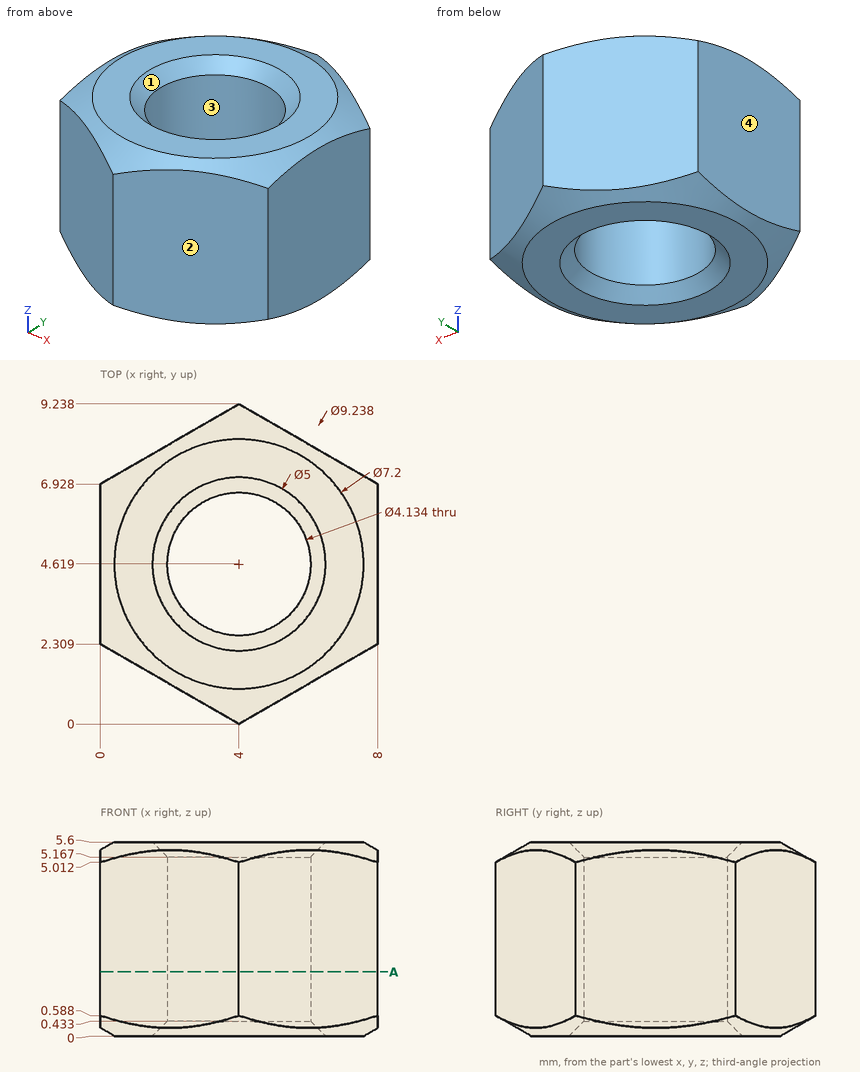
Geometry check sheet. Reference: drawing and pictorial views, mm from the part's lowest x, y, z. Give positions to 0.01 mm unless a question says otherwise; leave off trailing zeros. Write each loop counter-clockwise with the first axis right and the second up, starting at its lowest first coordinate (ties: lowest second). Pieces come first, ordered by that corner, then holes. Notation, with made-up numbers: M 85.25,46.5 L 142.25,46.5 A16 ccw 142.25,66.5 Z; hole C -35.75,46 d5. An arc over 180 degrees is marked long. Use CSV: the item, a comma, the result in double quotes.
1) Go/stop test with flat-tipped pins: pin 1 Ø1.5 at (x, z) = (1.5, 1) entering from +Y; pin 2 Ø1.5 at (x, z) = (3, 4.5) entering from -Y (1 decimal); pin 3 Ø2 at (x, z) = (2.5, 4.5) entering from -Y. Record where each tip stops, or that it passes through.
Final values:
pin 1,"y = 8.23"
pin 2,"y = 0.1"
pin 3,"y = 0.29"
2) Release check for a two-part mould opening along Y. For the marked faces 1, 2, 3 and 4 record: released by +Y, released by -Y, zero draft, split by the parting line, or undercut.
Final values:
face 1,"undercut"
face 2,"released by -Y"
face 3,"undercut"
face 4,"zero draft"
3) Material ranges on line 1 along X through (y, z) = (4.5, 1.05); line 2 along X through (y, z) = (6, 3.7); line 3 along X through (y, z) = (7.5, 2.55), recorded low to high.
Final values:
line 1,"0 to 1.94, 6.06 to 8"
line 2,"0 to 2.46, 5.54 to 8"
line 3,"0.99 to 7.01"
4) Cross-section at A-A (z = 1.85). Enter the section's corners in (x, y).
Final values:
outline,"M 0,2.31 L 4,0 L 8,2.31 L 8,6.93 L 4,9.24 L 0,6.93 Z; hole C 4,4.62 d4.13"
